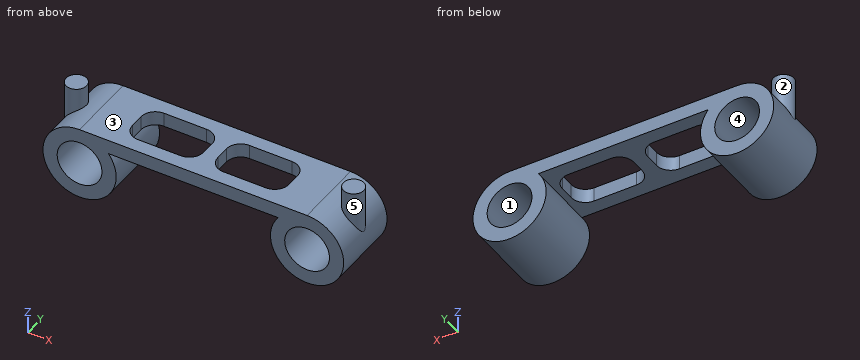
```python
from build123d import *

# Parameters (mm, degrees)
SKETCH1_R           = 3.15
BOSS_EXTRUDE1_DEPTH = 10
BOSS_EXTRUDE2_REACH = 27.562
SKETCH2_R           = 1.45
BOSS_EXTRUDE3_START = 2.5
SKETCH3_R           = 1.45
BOSS_EXTRUDE3_DEPTH = 2.5
CUT_EXTRUDE1_REACH  = 27.562
SKETCH4_W           = 10
SKETCH4_H           = 6
FILLET1_R           = 2


with BuildPart() as part:
    # Sketch1 → Boss-Extrude1 (new body)
    with BuildSketch(Plane(origin=(0, 0, 0), x_dir=(1, 0, 0), z_dir=(0, 1, 0))):
        with BuildLine():
            Line((11.925690243, -3.15), (-11.925690243, -3.15))
            ThreePointArc((-11.925690243, -3.15), (-18.269361144, 4.623040125), (-16, -5.15))
            Line((-16, -5.15), (16, -5.15))
            ThreePointArc((16, -5.15), (18.269361144, 4.623040125), (11.925690243, -3.15))
        make_face()
        with Locations(Location((-16, 0, 0), (0, 0, 270))):
            Circle(SKETCH1_R, mode=Mode.SUBTRACT)
        with Locations(Location((16, 0, 0), (0, 0, 270))):
            Circle(SKETCH1_R, mode=Mode.SUBTRACT)
    extrude(amount=BOSS_EXTRUDE1_DEPTH)

    # Sketch2 → Boss-Extrude2 (add, up to next)
    with BuildSketch(Plane.XY.offset(5.15), mode=Mode.PRIVATE) as boss_extrude2_sk1:
        with Locations((-19.5, 5)):
            Circle(SKETCH2_R)
    boss_extrude2_tool1 = extrude(boss_extrude2_sk1.sketch, amount=-BOSS_EXTRUDE2_REACH, mode=Mode.PRIVATE) - part.part
    # Sketch2 → Boss-Extrude2 (add, up to next)
    with BuildSketch(Plane.XY.offset(5.15), mode=Mode.PRIVATE) as boss_extrude2_sk2:
        with Locations((19.5, 5)):
            Circle(SKETCH2_R)
    boss_extrude2_tool2 = extrude(boss_extrude2_sk2.sketch, amount=-BOSS_EXTRUDE2_REACH, mode=Mode.PRIVATE) - part.part
    add(boss_extrude2_tool1.solids().sort_by_distance((-19.5, 5, 5.15))[0])
    add(boss_extrude2_tool2.solids().sort_by_distance((19.5, 5, 5.15))[0])

    # Sketch3 → Boss-Extrude3 (add)
    with BuildSketch(Plane.XY.offset(5.15).offset(BOSS_EXTRUDE3_START)):
        with Locations((-19.5, 5)):
            Circle(SKETCH3_R)
        with Locations((19.5, 5)):
            Circle(SKETCH3_R)
    extrude(amount=-BOSS_EXTRUDE3_DEPTH)

    # Sketch4 → Cut-Extrude1 (cut, up to next)
    with BuildSketch(Plane.XY.offset(5.15), mode=Mode.PRIVATE) as cut_extrude1_sk1:
        with Locations((-6, 5)):
            Rectangle(SKETCH4_W, SKETCH4_H)
    cut_extrude1_tool1 = extrude(cut_extrude1_sk1.sketch, amount=-CUT_EXTRUDE1_REACH, mode=Mode.PRIVATE) & part.part
    # Sketch4 → Cut-Extrude1 (cut, up to next)
    with BuildSketch(Plane.XY.offset(5.15), mode=Mode.PRIVATE) as cut_extrude1_sk2:
        with Locations((6, 5)):
            Rectangle(SKETCH4_W, SKETCH4_H)
    cut_extrude1_tool2 = extrude(cut_extrude1_sk2.sketch, amount=-CUT_EXTRUDE1_REACH, mode=Mode.PRIVATE) & part.part
    add(cut_extrude1_tool1.solids().sort_by_distance((-6, 5, 5.15))[0], mode=Mode.SUBTRACT)
    add(cut_extrude1_tool2.solids().sort_by_distance((6, 5, 5.15))[0], mode=Mode.SUBTRACT)

    # Fillet1
    fillet1_edges = [part.edges().sort_by_distance(p)[0] for p in [
        (-1, 8, 4.15),
        (-11, 8, 4.15),
        (-11, 2, 4.15),
        (-1, 2, 4.15),
        (11, 8, 4.15),
        (11, 2, 4.15),
        (1, 2, 4.15),
        (1, 8, 4.15),
    ]]
    fillet(fillet1_edges, radius=FILLET1_R)


solid = part.part
```
The listing builds one solid part. Answer for the finished solid, in the listing's coordinates (mm). Face numbers are marked on the shaded views. A direction names the side the tool comes from. Round coordinates to 2 decimals unless told otherwise and drop trailing zeros. Write each loop counter-clockwise with the first axis right and the second up, starting at its lowest first coordinate (ties: lowest second). Pieces come first, ordered by that corner, then holes. Notation, with made-up numbers: (46, 28.5) -> (90, 28.5) arc R12 ccw to (90, 44.5) -> close; hole circle Ø10 at (-39.5, 1). An arc over 180 degrees is marked (long way). Answer as a JSON object with one key per item and string values. Group by question number.
Q1. Each of these flat-tipped pins is pushed along its axis until it touches: pin 1 Ø1.6 at (y, z) = (4.5, 4.5) entering from +X; pin 2 Ø5 at (x, y) = (10.5, 1.5) entering from -Z; pin 3 Ø2 at (y, z) = (5, 3.5) entering from -X. Where does it stop, or does it pass through?
Q2. Which of the six approach directions +Z, -Z, +X, -X, +Y, -Y give full straight-line access (tool end or side, diameter ignored) to the marked faces 1 and 2?
Q3. Section D-D (z = 6.75) is taken. Write down the section's boundary in (x, y).
Q4. Determine the mould class of the marked faces 3, 4 and 5 for opening direction Z: pulls with the +Z half, pulls with the -Z half, needs draft (parallel to the pull), parting line crosses it, or undercut.
Q5. Section A-A (x = 4) is taken. Write down the section's boundary in (y, z), plus the area to 3 significant figures.
Q6. Straight lines are drawn through the part: line 1 along X through (y, z) = (4.75, 0); line 2 along X through (y, z) = (4.5, -1.5); line 3 along Z through (x, y) = (9.5, 8.25). For each, find the intervals that lie inside material, in ascending order.
Q7. Section B-B (z = 0) is taken. Write down the section's boundary in (x, y), plus the area to 3 significant figures.
Q8. Section C-C (y = 0.5) is taken. Write down the section's boundary in (x, z), plus the area to 3 significant figures.
Check values:
{
 "1": {"pin 1": "x = 20.95", "pin 2": "z = -4.19", "pin 3": "x = -20.95"},
 "2": {"face 1": "+Y, -Y", "face 2": "+Z"},
 "3": {"outline": "circle Ø2.9 at (-19.5, 5); circle Ø2.9 at (19.5, 5)"},
 "4": {"face 3": "pulls with the +Z half", "face 4": "undercut", "face 5": "needs draft"},
 "5": {"outline": "(0, 3.15) -> (2, 3.15) -> (2, 5.15) -> (0, 5.15) -> close; (8, 3.15) -> (10, 3.15) -> (10, 5.15) -> (8, 5.15) -> close", "area": "8.00 mm^2"},
 "6": {"line 1": "-21.15 to -19.15, -12.85 to -10.85, 10.85 to 12.85, 19.15 to 21.15", "line 2": "-20.93 to -18.77, -13.23 to -11.07, 11.07 to 13.23, 18.77 to 20.93", "line 3": "3.15 to 5.15"},
 "7": {"outline": "(-21.15, 0) -> (-19.15, 0) -> (-19.15, 10) -> (-21.15, 10) -> close; (-12.85, 0) -> (-10.85, 0) -> (-10.85, 10) -> (-12.85, 10) -> close; (10.85, 0) -> (12.85, 0) -> (12.85, 10) -> (10.85, 10) -> close; (19.15, 0) -> (21.15, 0) -> (21.15, 10) -> (19.15, 10) -> close", "area": "80.0 mm^2"},
 "8": {"outline": "(-16, 5.15) arc R5.15 ccw (long way) to (-11.93, 3.15) -> (11.93, 3.15) arc R5.15 ccw (long way) to (16, 5.15) -> close; hole circle Ø6.3 at (-16, 0); hole circle Ø6.3 at (16, 0)", "area": "157 mm^2"}
}
